Autodesk Inventor part; units mm, degrees
ref_plane "YZ Plane" through (0, 0, 0) normal (1, 0, 0) x (0, 1, 0)
ref_plane "XZ Plane" through (0, 0, 0) normal (0, 1, 0) x (-1, 0, 0)
ref_plane "XY Plane" through (0, 0, 0) normal (0, 0, 1) x (1, 0, 0)
sketch "Sketch1" plane through (0, 0, 0) normal (0, 0, 1) x (1, 0, 0)
  circle A0 centre (0, 0) radius 1.5
  circle A1 centre (0, 0) radius 3
  line L0 (0, 3) -> (28, 3)
  line L1 (28, 3) -> (28, -3)
  line L2 (28, -3) -> (0, -3)
  line L3 (0, -3) -> (0, 3)
  line L4 (28, 3) -> (10, 3)
  line L5 (10, 3) -> (10, 59)
  line L6 (10, 59) -> (28, 59)
  line L7 (28, 59) -> (28, 3)
  circle A2 centre (23.5, 28.5) radius 5.5
  circle A3 centre (18.553, 47) radius 6.25
  line L8 (23.5, 28.5) -> (18.553, 47) construction
  line L9 (23.5, 28.5) -> (10, 28.5) construction
  circle A4 centre (18.553, 38.5) radius 0.8
  circle A5 centre (25.9142, 51.25) radius 0.8
  circle A6 centre (11.1918, 51.25) radius 0.8
  line L10 (10, 59) -> (6, 59)
  line L11 (6, 59) -> (6, 45)
  line L12 (6, 45) -> (10, 45)
  line L13 (10, 45) -> (10, 59)
  line L14 (6, 45) -> (10, 41)
  line L15 (6, 45) -> (11.6569, 45) construction
  line L16 (28, 34.5) -> (31, 34.5)
  line L17 (31, 34.5) -> (31, 22.5)
  line L18 (31, 22.5) -> (28, 22.5)
  line L19 (28, 22.5) -> (28, 34.5)
  line L20 (31, 34.5) -> (28, 37.5)
  line L21 (31, 34.5) -> (35.2426, 34.5) construction
  line L22 (31, 22.5) -> (28, 19.5)
  line L23 (31, 22.5) -> (35.2426, 22.5) construction
  circle A7 centre (12.5, 7.5) radius 1.5
  circle A8 centre (17.5, 11.5) radius 1.25
  circle A9 centre (25, 10.5) radius 1.25
  line L24 (18.553, 47) -> (6, 47) construction
  line L25 (18.553, 38.5) -> (18.553, 47) construction
  dimension "d0" = 3
  dimension "d1" = 6
  dimension "d2" = 28
  dimension "d3" = 6
  dimension "d4" = 0
  dimension "d5" = 3
  dimension "d6" = 18
  dimension "d7" = 56
  dimension "d8" = 11
  dimension "d9" = 4.5
  dimension "d10" = 25.5
  dimension "d11" = 12.5
  dimension "d12" = 19.15
  dimension "d14" = 1.6
  dimension "d17" = 12
  dimension "d20" = 360
  dimension "d22" = 4
  dimension "d23" = 14
  dimension "d24" = 45
  dimension "d25" = 3
  dimension "d26" = 12
  dimension "d27" = 6
  dimension "d28" = 135
  dimension "d29" = 135
  dimension "d32" = 3
  dimension "d33" = 10.5
  dimension "d34" = 2.5
  dimension "d35" = 2.5
  dimension "d36" = 14.5
  dimension "d37" = 7.5
  dimension "d38" = 2.5
  dimension "d39" = 15
  dimension "d40" = 13.5
  dimension "d60" = 8.5
  dimension "d61" = 270
extrude "Extrusion1" add sketch "Sketch1" along normal blind 5 contours A0 L3 A1 | A0 L3 A1 | L0 L1 L2 A1 | L5 L6 L7 A2 L0 | L14 L12 L5 | L7 L18 L22 | L12 L11 L10 L5 | L7 A2 L16 L17 L18 | L16 L7 L20
fillet "Fillet1" radius 2 1 edges at (28, -3, 2.5)
fillet "Fillet2" radius 2 1 edges at (10, 3, 2.5)
sketch "Sketch2" plane through (0, 0, 5) normal (0, 0, 1) x (1, 0, 0)
  line L0 (28, -1) -> (28, 19.5)
  line L1 (0, -3) -> (26, -3)
  line L2 (28, -1) -> (28, 19.5)
  line L3 (28, 20.75) -> (15.25, 20.75)
  line L4 (15.25, 20.75) -> (15.25, 0.75)
  line L5 (15.25, 0.75) -> (28, 0.75)
  line L6 (28, 0.75) -> (28, 20.75)
  line L7 (28, 19.5) -> (31, 22.5)
  line L8 (28, 20.75) -> (29.25, 20.75)
  line L9 (28, 19.5) -> (31, 22.5)
  point P0 (0, 0)
  point P1 (28, 19.5)
  point P2 (28, 19.5)
  dimension "d43" = 12.75
  dimension "d44" = 20
  dimension "d45" = 23.75
extrude "Extrusion2" cut sketch "Sketch2" against normal blind 4
sketch "Sketch3" plane through (6, 59, 0) normal (0, 1, 0) x (1, 0, 0)
  circle A0 centre (3, -2.5) radius 1.5
  line L0 (22, 0) -> (0, 0)
  line L1 (0, 0) -> (0, -5)
  line L2 (22, -5) -> (0, -5)
  line L3 (22, 0) -> (22, -5)
  circle A1 centre (19, -2.5) radius 1.5
  dimension "d48" = 3
  dimension "d49" = 3
  dimension "d50" = 2.5
  dimension "d51" = 2.5
  dimension "d52" = 3
  dimension "d53" = 3
extrude "Extrusion3" cut sketch "Sketch3" against normal blind 6 contours A0 | A1
thread "Thread1"
thread "Thread2"
sketch "Sketch5" plane through (0, 0, 5) normal (0, 0, 1) x (1, 0, 0)
  circle A0 centre (18.553, 38.5) radius 0.8
  circle A1 centre (11.1918, 51.25) radius 0.8
  circle A2 centre (25.9142, 51.25) radius 0.8
  circle A3 centre (18.553, 38.5) radius 1.5
  circle A4 centre (11.1918, 51.25) radius 1.5
  circle A5 centre (25.9142, 51.25) radius 1.5
  point P0 (0, 0)
  dimension "d62" = 3
  dimension "d63" = 3
  dimension "d64" = 3
extrude "Extrusion4" cut sketch "Sketch5" against normal blind 3 contours A0 | A1 | A2 | A3 | A4 | A5
properties part number "PartA"
Design review of the part built by this model. Coordinates are the model's own, in mm. A direction names the side the tool comes from. Give positions to 0.01 mm unless a question says otherwise; leave off trailing zeros. Loops run counter-clockwise (first coordinate to the right, second up) from the corner with the lowest first, then second, coordinate; pieces in that order, holes last. Notation, with made-up numbers: M 1.25,47 L 33.25,47 A20 ccw 33.25,72 Z; hole C -38.5,-11 d3. An arc over 180 degrees is marked long. One line per question, with ' | ' between items. Start each with the question number.
1. The part is to be moulded in two halves that separate along Z. For faces 1 (the face through (23.5, 56.04, 2.43)), 2 (the face through (-1.5, -0.07, 2.46)), 3 (the face through (18, 35, 5)), say which applies: released by +Z, released by -Z, zero draft, split by the parting line, or undercut.
2. Add section B-B (y = 7.5). Write out the cut boundary in (x, z).
3. Insertion check: P1, Ø7, axis at x = 23, y = 12, coming from the +Z side; P2, Ø3, axis at x = 22, y = 13.5, coming from the -Z side; P3, Ø2, axis at y = 11.5, z = 3, coming from the +X side; P4, Ø2.5, axis at x = 11.19, y = 51.25, coming from the +Z side. Each pin has a flat end and moves straight along its axis. Give the tip position at first contact, or say it passes through.
4. Add section D-D (y = 0). Write out the cut boundary in (x, z), plus the area to 3 significant figures.
5. For faces 4 (the face through (15.25, 11, 3)), 5 (the face through (19.25, 37.17, 3.52)), 6 (the face through (28, 48, 2)), 7 (the face through (9, 53, 2)), list the 3-axis set-ups (+Z, -Z, +X, -X, +Y, -Y) from which the entire face can be reached by the end or side of a thin tool; tool diameter is ignored.
6. Add section A-A (y = 38.5). Write out the cut boundary in (x, z).
7. Add section C-C (x = 4.5). Write out the cut boundary in (y, z).
8. To check wall thickness, follow L1, parallel to X at y = 54.45, z = 2.5; L2, parallel to X at y = 38.5, z = 1.35; L3, parallel to Y at x = 27.5, z = 2.7. State the ranges of each line that lie inside material, in increasing order.
Worked out:
1) face 1: undercut | face 2: zero draft | face 3: released by +Z
2) outline: M 10,0 L 11,0 L 11,5 L 10,5 Z; M 14,0 L 28,0 L 28,1 L 15.25,1 L 15.25,5 L 14,5 Z
3) P1: stops at z = 1 | P2: stops at z = 0 | P3: stops at x = 15.25 | P4: stops at z = 2
4) outline: M -3,0 L -1.5,0 L -1.5,5 L -3,5 Z; M 1.5,0 L 28,0 L 28,5 L 1.5,5 Z | area: 140 mm²
5) face 4: +Z, +X | face 5: +Z | face 6: +Z, -Z, +X, +Y | face 7: +Y
6) outline: M 10,0 L 17.75,0 L 17.75,2 L 17.05,2 L 17.05,5 L 10,5 Z; M 19.35,0 L 28,0 L 28,5 L 20.05,5 L 20.05,2 L 19.35,2 Z
7) outline: M -3,0 L 3,0 L 3,5 L -3,5 Z
8) L1: x = 6 to 7.5, 10.5 to 23.5, 26.5 to 28 | L2: x = 10 to 17.75, 19.35 to 28 | L3: y = -2.32 to 0.75, 20.75 to 24.73, 32.27 to 59
